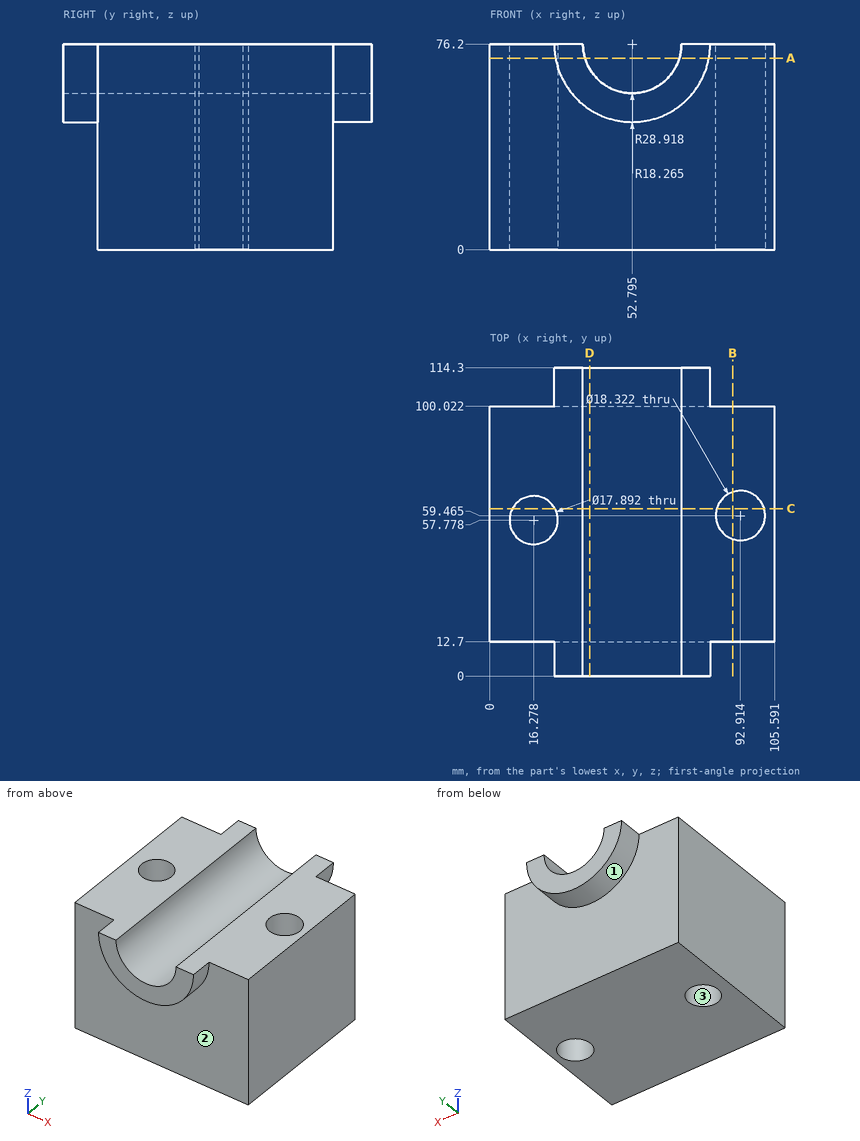
Could you check a few things on this drawing? It's one solid part, dimensions in mm from its lowest x, y, z. Give positions to 0.01 mm unless a question says otherwise; leave off trailing zeros. Write each loop counter-clockwise with the first axis right and the second up, starting at its lowest first coordinate (ties: lowest second). Pieces come first, ordered by that corner, then holes. Notation, with made-up numbers: (35, 34.25) -> (52, 34.25) arc R25 cw to (52, 59.25) -> close; hole circle Ø6 at (13.25, -17.75). An arc over 180 degrees is marked (long way). Answer as CSV lines item,"result". Start each with the question number.
(1) If we section it at A-A, the plane z = 71: Write out the boundary of the cut face in (x, y) (1 decimal), and give its area (3 significant figures).
(2) If we mould it in two halves opening along Y, with no side actions, what happens to the marked faces 1, 2 and 3? For each: +Y half, -Y half, draft (parallel to the pull), parting line (faces both ways), or undercut.
(3) If we section it at C-C, the plane y = 62: Write out the boundary of the cut face in (x, z) (1 decimal).
(4) If we section it at B-B, the plane x = 90: Write out the boundary of the cut face in (y, z), and give its area (3 significant figures).
(5) I'm going to push flat-ended pins straight in: pin 1 Ø2 at (x, z) = (49, 38) entering from -Y; pin 2 Ø23 at (x, z) = (63.5, 35.5) entering from +Y. Where does each tip first touch, or does it pass through?
(6) If we section it at D-D, the plane x = 37: Write out the boundary of the cut face in (y, z).
(7) Please list where these lines run through material, in increasing order: line 1 (X direction, y = 54, z = 37.5) (1 decimal); line 2 (X direction, y = 63, z = 38) (1 decimal); line 3 (Y direction, x = 29, z = 23.5).
Answer list:
1,outline,"(0, 12.7) -> (24.3, 12.7) -> (24.3, 0) -> (35.3, 0) -> (35.3, 114.3) -> (24.3, 114.3) -> (24.3, 100) -> (0, 100) -> close; (70.3, 0) -> (81.2, 0) -> (81.2, 12.7) -> (105.6, 12.7) -> (105.6, 100) -> (81.2, 100) -> (81.2, 114.3) -> (70.3, 114.3) -> close; hole circle Ø17.9 at (16.3, 57.8); hole circle Ø18.3 at (92.9, 59.5)"
1,area,"6,240 mm^2"
2,face 1,"draft"
2,face 2,"-Y half"
2,face 3,"undercut"
3,outline,"(0, 0) -> (8.4, 0) -> (8.4, 76.2) -> (0, 76.2) -> close; (24.2, 0) -> (84.1, 0) -> (84.1, 76.2) -> (71.1, 76.2) arc R18.3 cw to (34.5, 76.2) -> (24.2, 76.2) -> close; (101.7, 0) -> (105.6, 0) -> (105.6, 76.2) -> (101.7, 76.2) -> close"
4,outline,"(12.7, 0) -> (50.78, 0) -> (50.78, 76.2) -> (12.7, 76.2) -> close; (68.15, 0) -> (100.02, 0) -> (100.02, 76.2) -> (68.15, 76.2) -> close"
4,area,"5,330 mm^2"
5,pin 1,"y = 12.7"
5,pin 2,"y = 100.02"
6,outline,"(0, 51.98) -> (12.7, 51.98) -> (12.7, 0) -> (100.02, 0) -> (100.02, 51.98) -> (114.3, 51.98) -> (114.3, 67.03) -> (0, 67.03) -> close"
7,line 1,"0 to 8.2, 24.4 to 85.6, 100.3 to 105.6"
7,line 2,"0 to 9, 23.5 to 84.5, 101.4 to 105.6"
7,line 3,"12.7 to 100.02"
